Verification items for this drawing (mm, ordinates from the low corner). Round coordinates to 2 decimals unless told otherwise and drop trailing zeros. Loops run counter-clockwise (first coordinate to the right, second up) from the corner with the lowest first, then second, coordinate; pieces in that order, holes last. Notation, with made-up numbers: M 70,29 L 124,29 A30 ccw 124,66 Z; hole C 37.25,87 d9. An arc over 180 degrees is marked long. Write item = value, one per line. Start each with the question number.
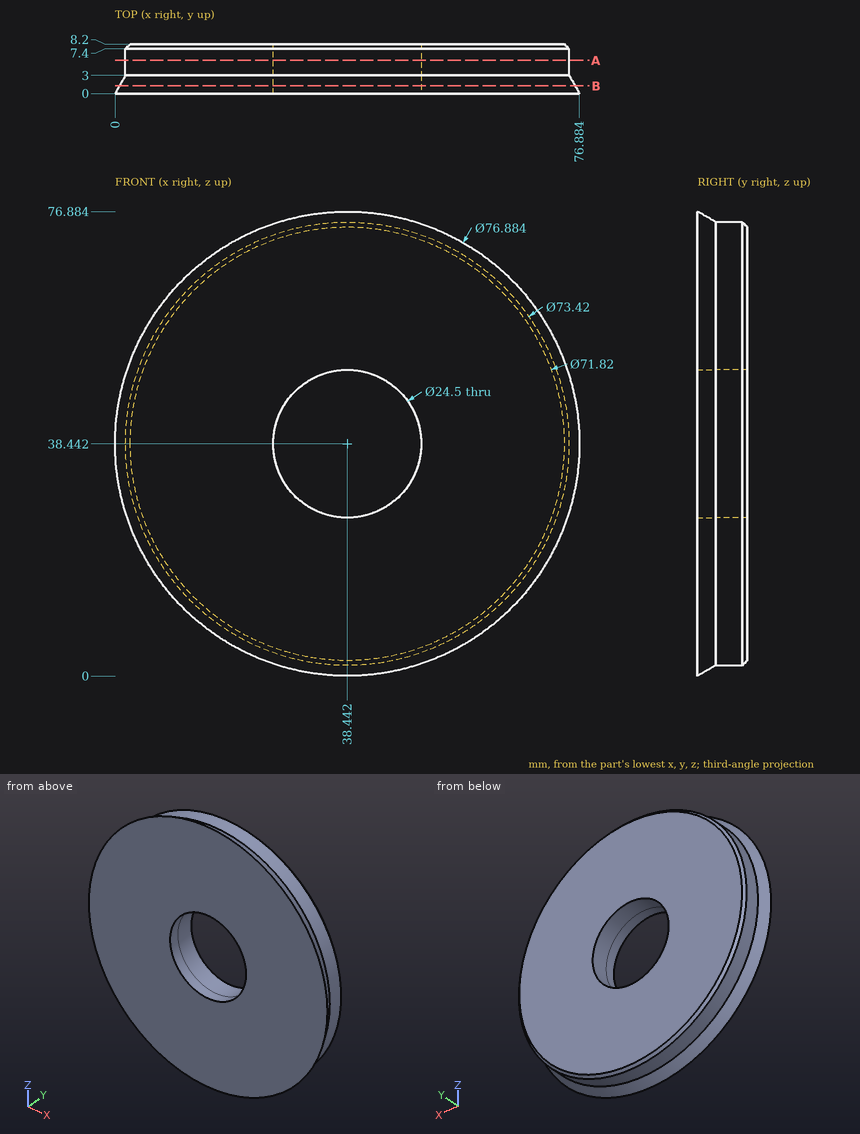
1. Section check B-B, the plane y = 1.25. Enter the section's corners in (x, z), and give its area (3 significant figures).
2. Thickness scan on line 1 (X direction, y = 1.25, z = 28) (1 decimal); line 2 (X direction, y = 4.5, z = 42) (1 decimal); line 3 (X direction, y = 3.5, z = 58.5). Record the ranges inside material, lowest first.
3. Gauge pin test, flat ends, axial feed: P1, Ø3, axis at y = 1.5, z = 59, coming from the +X side; P2, Ø1.5, axis at y = 5.5, z = 17, coming from the -X side; P3, Ø2, axis at x = 33, y = 2.5, coming from the +Z side; P4, Ø14.5, axis at x = 38.44, z = 38.44, coming from the -Y side. Record the tip position at first contact, or that the pin passes through.
4. Section check A-A, the plane y = 5.5. Enter the section's corners in (x, z), and give its area (3 significant figures).
Computed values:
q1.outline = C 38.44,38.44 d75.44; hole C 38.44,38.44 d24.5
q1.area = 4,000 mm2
q2.line_1 = 2.2 to 32, 44.8 to 74.7
q2.line_2 = 1.9 to 26.7, 50.2 to 75
q2.line_3 = 7.7 to 69.19
q3.P1 = 71.28
q3.P2 = 8.12
q3.P3 = 75.64
q3.P4 = through
q4.outline = C 38.44,38.44 d73.42; hole C 38.44,38.44 d24.5
q4.area = 3,760 mm2
